Work out the finished part from the listing and answer in its coordinate system (mm). A direction names the side the tool comes from. Round coordinates to 2 decimals unless told otherwise and drop trailing zeros. Loops run counter-clockwise (first coordinate to the right, second up) from the corner with the lowest first, then second, coordinate; pieces in that order, holes last. Notation, with made-up numbers: M 29,13 L 75,13 A20 cw 75,36 Z; hole C 40.25,7 d11. An arc over 180 degrees is marked long. One line per item, written item: value.
```python
from build123d import *

# Parameters (mm, degrees)
F0_R     = 11.90906
F1_DEPTH = 25
F2_COUNT = 12


with BuildPart() as f1:
    # F0 (on Front) → F1 (new body)
    with BuildSketch(Plane.XZ):
        with BuildLine():
            ThreePointArc((-4.4772, 26.540564), (-0.095682, 26.927299), (4.290206, 26.593761))
            ThreePointArc((4.290206, 26.593761), (4.28911, 29.570632), (3.706133, 32.489861))
            ThreePointArc((3.706133, 32.489861), (2.632484, 35.065209), (1.07088, 37.377466))
            ThreePointArc((1.07088, 37.377466), (-0.312037, 38.054077), (-1.667357, 37.323755))
            ThreePointArc((-1.667357, 37.323755), (-3.137083, 34.952037), (-4.108913, 32.336566))
            ThreePointArc((-4.108913, 32.336566), (-4.573289, 29.456371), (-4.4772, 26.540564))
        make_face()
        with BuildLine():
            ThreePointArc((-4.4772, 26.540564), (-17.244829, -20.469915), (26.927793, 0.067293))
            ThreePointArc((26.927793, 0.067293), (20.499082, 17.503705), (4.290206, 26.593761))
            ThreePointArc((4.290206, 26.593761), (-0.095682, 26.927299), (-4.4772, 26.540564))
        make_face()
        with Locations((0.067293, 0.067293)):
            Circle(F0_R, mode=Mode.SUBTRACT)
    extrude(amount=F1_DEPTH)

    # F2: F1 ×12 about axis
    f2_axis = Axis((0.067293, 0, 0.067293), (0, 1, 0))


with BuildPart() as f1_1:
    add(f1.part)
    for i in range(1, F2_COUNT):
        add(f1.part.rotate(f2_axis, i * 360 / F2_COUNT))


solid = f1_1.part
```
1) The mould has two halves that part along Z. Classify faces 1 (the face through (10.766, -12.325, 27.873)), 2 (the face through (29.53, -12.32, -4.16)), 3 (the face through (-25.845, -12.325, -7.007)), 4 (the face through (29.05, -12.32, -19.65)): +Z half, -Z half, draft (parallel to the pull), parting line (faces both ways), or undercut.
Check values:
face 1: +Z half
face 2: undercut
face 3: undercut
face 4: -Z half
2) Find section C-C (z = 15.5). Give the vertices of the cut face in (x, y).
Check values:
outline: M -32.23,-25 L 31.75,-25 L 31.75,0 L -32.23,0 Z
3) For faces 5 (the face through (31.9, -12.32, -14.63)), 6 (the face through (-4.16, -12.32, -29.39)), 7 (the face through (-27.739, -12.325, 10.766)), 8 (the face through (-18.617, -12.325, -33.009)), 9 (the face through (-11, -12.32, 27.69)), determine the directions among +Z, -Z, +X, -X, +Y, -Y from which every point of the face is accessible in a straight line to the end or side of a thin tool.
Check values:
face 5: +X, +Y, -Y
face 6: +Y, -Y
face 7: -X, +Y, -Y
face 8: -Z, +Y, -Y
face 9: +Z, +Y, -Y
4) Find the intervals of material crossed by probe 1 along Z at (x, y) = (-30.5, -11.25); probe 2 along Z at (x, y) = (18.5, -13.25) (3 decimals); probe 3 along X at (y, z) = (-7.75, -29.5), in increasing order. Write a range as from..to.
Check values:
probe 1: -20.15..-13.76, -4.45..4.15, 13.14..19.75
probe 2: -32.883..-22.525, -19.47..19.605, 23.562..33.26
probe 3: -19.66..-12.01, -4.15..4.7, 12.78..20.32
5) Each of these flat-tipped pins is pushed along its axis until it touches: pin 1 (1.5 mm diameter, centred on x = 18, y = -9.5, fed in from +Z); pin 2 (8 mm diameter, centred on x = 22, y = -7.5, fed in from -Z); pin 3 (3 mm diameter, centred on x = -22.5, z = 1, fed in from +Y); pin 4 (14.5 mm diameter, centred on x = 0.07, z = 0.07, fed in from -Y). Where does it stop, or does it pass through?
Check values:
pin 1: z = 33.36
pin 2: z = -32.88
pin 3: y = 0
pin 4: through
6) Find section B-B (x = 15). Give the vertices of the cut face in (y, z).
Check values:
outline: M -25,-31.3 L 0,-31.3 L 0,32.05 L -25,32.05 Z
7) Find section A-A (x = -6.5). Give the vertices of the cut face in (y, z), then the cut area to 3 significant figures.
Check values:
outline: M -25,-25.98 L 0,-25.98 L 0,-9.87 L -25,-9.87 Z; M -25,10 L 0,10 L 0,26.11 L -25,26.11 Z
area: 806 mm2
